from build123d import *

# Parameters (mm, degrees)
F0_R     = 2.5
F1_DEPTH = 5
F2_SIZE  = 4.99999


# Not quite as in the source:
# - a fillet or chamfer is up to 0.001 mm smaller than in the source, because OpenCascade refuses the exact size


with BuildPart() as f1:
    # F0 (on Right) → F1 (new body)
    with BuildSketch(Plane.YZ):
        Polygon((-10, 0), (10, 0), (10, 40), (20, 40), (20, 60), (-20, 60), (-20, 40), (-10, 40), align=None)
        with Locations((0, 10)):
            Circle(F0_R, mode=Mode.SUBTRACT)
        with Locations((-10, 50)):
            Circle(F0_R, mode=Mode.SUBTRACT)
        with Locations((0, 30)):
            Circle(F0_R, mode=Mode.SUBTRACT)
        with Locations((10, 50)):
            Circle(F0_R, mode=Mode.SUBTRACT)
    extrude(amount=F1_DEPTH)

    # F2 (size 5 in the source; OpenCascade refuses exactly that, so slightly less here)
    f2_edges = [f1.edges().sort_by_distance(p)[0] for p in [
        (2.5, 10, 40),
        (2.5, 20, 40),
        (2.5, 20, 60),
        (2.5, 10, 0),
        (2.5, -10, 0),
        (2.5, -10, 40),
        (2.5, -20, 40),
        (2.5, -20, 60),
    ]]
    chamfer(f2_edges, length=F2_SIZE)


solid = f1.part
Here's how the part is built. I have some questions about the finished solid (model axes, mm). A direction names the side the tool comes from. Give positions to 0.01 mm unless a question says otherwise; leave off trailing zeros. Write each loop counter-clockwise with the first axis right and the second up, starting at its lowest first coordinate (ties: lowest second). Pieces come first, ordered by that corner, then holes. Notation, with made-up numbers: (-34, 53.25) -> (-2, 53.25) arc R28 cw to (-2, 89.25) -> close; hole circle Ø5 at (26.25, -32). An arc over 180 degrees is marked (long way). Use one line per item in the form item = value. Start each with the question number.
1. Imagine slicing it at B-B on y = 0. List the corners of the cut face in (x, z) for me, plus the area to 3 significant figures.
2. Imagine slicing it at C-C on z = 50. List the corners of the cut face in (x, y) for me.
3. Thinking about a two-plate mould opening in Y: for faces 3 (the face through (2.46, 1.34, 32.11)), 4 (the face through (2.46, -0.54, 7.56)), 5 (the face through (2, 0, 0)), 6 (the face through (2, 10, 20)), which applies, +Y half, -Y half, draft (parallel to the pull), parting line (faces both ways), or undercut?
4. On a 3-axis mill with a long thin cutter (end or side, diameter ignored), from which of +Z, -Z, +X, -X, +Y, -Y can I reach the whole of each face in a straight line? I mean faces 1 (the face through (2, -10, 20)), 2 (the face through (2, 18, 43)). Say none if no direction works.
5. If I drill on L1, parallel to Z at x = 4, y = 0; L2, parallel to Z at x = 2.5, y = -0.5; L3, parallel to Z at x = 1.45, y = -15, over which ranges is the centre line in solid material (lowest first)?
6. Imagine slicing it at D-D on x = 3.8. State how many separate pieces and enclosed holes the cut face has, plus the area to 3 significant figures.
7. Imagine slicing it at A-A on z = 30. List the corners of the cut face in (x, y) for me.
8. Will these pins go through, and if not, where does the flat tip stop? pin 1 Ø3 at (x, z) = (2, 22.5) entering from +Y; pin 2 Ø6 at (y, z) = (0, 30) entering from -X; pin 3 Ø4 at (y, z) = (10, 50) entering from +X; pin 4 Ø1.5 at (x, z) = (3.5, 40) entering from -Y.
Entries:
q1.outline = (0, 0) -> (5, 0) -> (5, 7.5) -> (0, 7.5) -> close; (0, 12.5) -> (5, 12.5) -> (5, 27.5) -> (0, 27.5) -> close; (0, 32.5) -> (5, 32.5) -> (5, 60) -> (0, 60) -> close
q1.area = 250 mm²
q2.outline = (0, -20) -> (5, -20) -> (5, -12.5) -> (0, -12.5) -> close; (0, -7.5) -> (5, -7.5) -> (5, 7.5) -> (0, 7.5) -> close; (0, 12.5) -> (5, 12.5) -> (5, 20) -> (0, 20) -> close
q3.face_3 = undercut
q3.face_4 = undercut
q3.face_5 = draft
q3.face_6 = +Y half
q4.face_1 = -Z, +X, -X, -Y
q4.face_2 = -Z, +X, -X, +Y
q5.L1 = 0 to 7.5, 12.5 to 27.5, 32.5 to 60
q5.L2 = 0 to 7.55, 12.45 to 27.55, 32.45 to 60
q5.L3 = 40 to 60
q6.separate_pieces = 1
q6.enclosed_holes = 4
q6.area = 1,470 mm²
q7.outline = (0, -10) -> (5, -10) -> (5, -2.5) -> (0, -2.5) -> close; (0, 2.5) -> (5, 2.5) -> (5, 10) -> (0, 10) -> close
q8.pin_1 = 10
q8.pin_2 = 0
q8.pin_3 = through
q8.pin_4 = -15.75
